```python
from build123d import *

# Parameters (mm, degrees)
SKETCH1_R           = 3.5
BOSS_EXTRUDE1_DEPTH = 3


with BuildPart() as part:
    # Sketch1 → Boss-Extrude1 (new body)
    with BuildSketch(Plane(origin=(0, 0, 0), x_dir=(1, 0, 0), z_dir=(0, 1, 0))):
        with BuildLine():
            Line((-4.808650437, 65.398437121), (-13.750473528, 53.416033622))
            ThreePointArc((-13.750473528, 53.416033622), (-14.783823427, 51.435125012), (-15.140381351, 49.229523647))
            Line((-15.140381351, 49.229523647), (-15.140381351, 0))
            Line((-15.140381351, 0), (-15.140381351, -49.229523647))
            ThreePointArc((-15.140381351, -49.229523647), (-14.783823427, -51.435125012), (-13.750473528, -53.416033622))
            Line((-13.750473528, -53.416033622), (-4.808650437, -65.398437121))
            ThreePointArc((-4.808650437, -65.398437121), (3.588437121, -66.618650437), (4.808650437, -58.221562879))
            Line((4.808650437, -58.221562879), (-3.140381351, -47.569539757))
            Line((-3.140381351, -47.569539757), (-3.140381351, 0))
            Line((-3.140381351, 0), (-3.140381351, 47.569539757))
            Line((-3.140381351, 47.569539757), (4.808650437, 58.221562879))
            ThreePointArc((4.808650437, 58.221562879), (3.588437121, 66.618650437), (-4.808650437, 65.398437121))
        make_face()
        with Locations(Location((0, 61.81, 0), (0, 0, 270))):
            Circle(SKETCH1_R, mode=Mode.SUBTRACT)
        with Locations(Location((0, -61.881, 0), (0, 0, 270))):
            Circle(SKETCH1_R, mode=Mode.SUBTRACT)
    extrude(amount=BOSS_EXTRUDE1_DEPTH)


solid = part.part
```
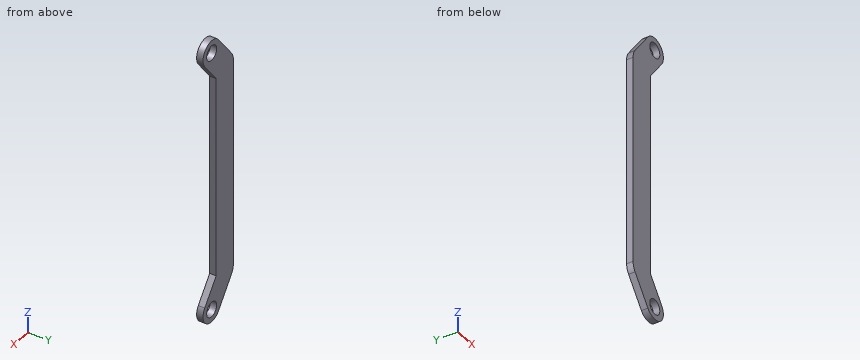
Source: CAD feature listing. Evaluate the final solid. Frame: model axes, mm. Coordinates: 2 decimals unless noted, no trailing zeros. Write each loop counter-clockwise with the first axis right and the second up, starting at its lowest first coordinate (ties: lowest second). Pieces come first, ordered by that corner, then holes. Notation, with made-up numbers: (41.25, 48) -> (98.25, 48) arc R28 ccw to (98.25, 74) -> close; hole circle Ø7 at (35, 2.25). An arc over 180 degrees is marked (long way). Return JSON: item names as keys, results as strings. Group by question number.
1) Section query B-B, the plane x = 0. Return loops of the section in (y, z), plus the area to 3 significant figures.
2) Section query C-C, the plane z = -61.81. Return loops of the section in (x, y).
3) Contact query for flat-ended pins moving along their axis: P1, Ø3, axis at x = -3.5, z = 20.5, coming from the -Y side; P2, Ø1.5, axis at y = 1, z = -4, coming from the +X side. Output: stop coordinate, or through.
4) Ray query, line 1 along Z through (x, y) = (3, 0.95); line 2 along X through (y, z) = (0.6, -44.5); line 3 along X through (y, z) = (2.15, -61.81). Return the intervals inside material, ascending.
5) Section query D-D, the plane z = 23.5. Return loops of the section in (x, y), plus the area to 3 significant figures.
6) Section query A-A, the plane y = 1.95. Return loops of the section in (x, z), plus the area to 3 significant figures.
From the geometry:
{
 "1": {"outline": "(0, -67.81) -> (3, -67.81) -> (3, -65.31) -> (0, -65.31) -> close; (0, -58.31) -> (3, -58.31) -> (3, -51.78) -> (0, -51.78) -> close; (0, 51.78) -> (3, 51.78) -> (3, 58.38) -> (0, 58.38) -> close; (0, 65.38) -> (3, 65.38) -> (3, 67.81) -> (0, 67.81) -> close", "area": "54.2 mm²"},
 "2": {"outline": "(-7.49, 0) -> (-3.5, 0) -> (-3.5, 3) -> (-7.49, 3) -> close; (3.5, 0) -> (6, 0) -> (6, 3) -> (3.5, 3) -> close"},
 "3": {"P1": "y = 0", "P2": "x = -3.14"},
 "4": {"line 1": "-67.01 to -63.61, -60.01 to -55.8, 55.8 to 60.08, 63.68 to 67.01", "line 2": "-15.14 to -3.14", "line 3": "-7.49 to -3.5, 3.5 to 6"},
 "5": {"outline": "(-15.14, 0) -> (-3.14, 0) -> (-3.14, 3) -> (-15.14, 3) -> close", "area": "36.0 mm²"},
 "6": {"outline": "(-15.14, -49.23) arc R7 ccw to (-13.75, -53.42) -> (-4.81, -65.4) arc R6 ccw to (4.81, -58.22) -> (-3.14, -47.57) -> (-3.14, 47.57) -> (4.81, 58.22) arc R6 ccw to (-4.81, 65.4) -> (-13.75, 53.42) arc R7 ccw to (-15.14, 49.23) -> close; hole circle Ø7 at (0, -61.81); hole circle Ø7 at (0, 61.88)", "area": "1,590 mm²"}
}
